```python
from build123d import *

# Parameters (mm, degrees)
TORUS001002001_R  = 1
CYLINDER002_R     = 10.9
CYLINDER002_DEPTH = 10.5
CYLINDER001_R     = 10.4
CYLINDER001_DEPTH = 130
CYLINDER_R        = 12.5
CYLINDER_DEPTH    = 130
FILLET_R          = 0.5


with BuildPart() as torus001002001:
    # Torus001002001 → Torus001002001 (revolve)
    with BuildSketch(Plane(origin=(0, 0, 80), x_dir=(1, 0, 0), z_dir=(0, -1, 0))):
        with Locations((13, 0)):
            Circle(TORUS001002001_R)
    revolve(axis=Axis((0, 0, 80), (0, 0, 1)))


with BuildPart() as cylinder002:
    # Cylinder002 → Cylinder002 (new body)
    with BuildSketch(Plane.XY.offset(119.5)):
        Circle(CYLINDER002_R)
    extrude(amount=CYLINDER002_DEPTH)


with BuildPart() as cylinder001:
    # Cylinder001 → Cylinder001 (new body)
    with BuildSketch(Plane.XY):
        Circle(CYLINDER001_R)
    extrude(amount=CYLINDER001_DEPTH)


with BuildPart() as fillet_body:
    # Cylinder → Cylinder (new body)
    with BuildSketch(Plane.XY):
        Circle(CYLINDER_R)
    extrude(amount=CYLINDER_DEPTH)

    # Cut: cut Cylinder001
    add(cylinder001.part, mode=Mode.SUBTRACT)

    # Cut001: cut Cylinder002
    add(cylinder002.part, mode=Mode.SUBTRACT)

    # Cut002: cut Torus001002001
    add(torus001002001.part, mode=Mode.SUBTRACT)

    # Fillet
    fillet_edges = [fillet_body.edges().sort_by_distance(p)[0] for p in [
        (-10.9, 0, 130),
    ]]
    fillet(fillet_edges, radius=FILLET_R)


solid = fillet_body.part
```
The listing builds one solid part. Answer for the finished solid, in the listing's coordinates (mm). Coordinates: 2 decimals unless noted, no trailing zeros. Write each loop counter-clockwise with the first axis right and the second up, starting at its lowest first coordinate (ties: lowest second). Pieces come first, ordered by that corner, then holes. Notation, with made-up numbers: M 26,40.5 L 76,40.5 A25 ccw 76,62.5 Z; hole C 80,84 d11. An arc over 180 degrees is marked long. Use a Markdown table: item, result. Add a question column.
1. Straight lines are drawn through the part: line 1 along Y through (x, z) = (0, 123); line 2 along Y through (x, z) = (0, 43); line 3 along X through (y, z) = (-4, 15). For each, find the intervals that lie inside material, in ascending order. Write a range as [from, to].
2. Section C-C (z = 83.5) is taken. Give the vertices of the cut face in (x, y), plus the area to 3 significant figures.
3. Section A-A (x = 0) is taken. Give the vertices of the cut face in (y, z), plus the area to 3 significant figures.
4. Given P1, Ø12, axis at x = 1.5, y = 0, coming from the +Z side; P2, Ø2, axis at x = -5, z = 63, coming from the -Y side; P3, Ø3, axis at y = -6, z = 104.5, coming from the +X side; P4, Ø4, axis at y = 7.5, z = 59.5, coming from the +X side (3 decimals), each flat-ended and moving along its own axis, determine where each tip first touches the part or whether it passes through.
5. For a pull along Y with two mould halves and no side action, classify faces 1 (the flat face through (4, -11, 130)), 2 (the cylindrical face through (10.4, 3.27, 124.43)), 3 (the cylindrical face through (11.923, 3.755, 105.089)) as +Y half, -Y half, draft (parallel to the pull), parting line (faces both ways), or undercut.
Data:
| question | item | result |
|---|---|---|
| 1 | line 1 | y = [-12.5, -10.9], [10.9, 12.5] |
| 1 | line 2 | y = [-12.5, -10.4], [10.4, 12.5] |
| 1 | line 3 | x = [-11.84, -9.6], [9.6, 11.84] |
| 2 | outline | C 0,0 d25; hole C 0,0 d20.8 |
| 2 | area | 151 mm2 |
| 3 | outline | M -12.5,0 L -10.4,0 L -10.4,119.5 L -10.9,119.5 L -10.9,129.5 A0.5 ccw -11.4,130 L -12.5,130 L -12.5,80.87 A1 cw -12.5,79.13 Z; M 10.4,0 L 12.5,0 L 12.5,79.13 A1 cw 12.5,80.87 L 12.5,130 L 11.4,130 A0.5 ccw 10.9,129.5 L 10.9,119.5 L 10.4,119.5 Z |
| 3 | area | 534 mm2 |
| 4 | P1 | passes through |
| 4 | P2 | stops at y = -11.84 |
| 4 | P3 | stops at x = 11.66 |
| 4 | P4 | stops at x = 11.225 |
| 5 | face 1 | draft |
| 5 | face 2 | undercut |
| 5 | face 3 | parting line |
